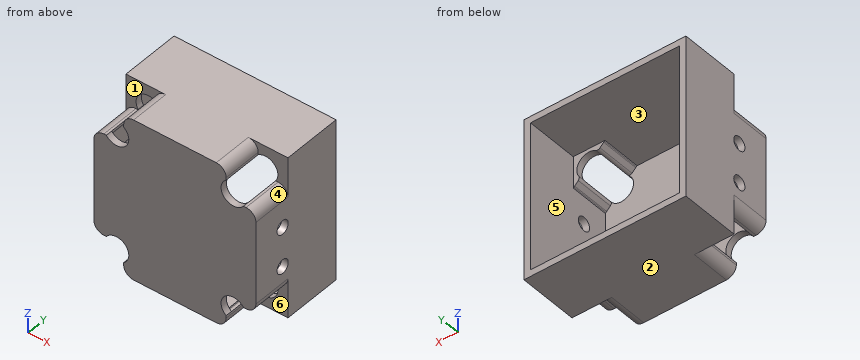
```python
from build123d import *

# Parameters (mm, degrees)
EXTRUDE_1_DEPTH          = 12
EXTRUDE_START            = 2
EXTRUDE_2_DEPTH          = 2
SKETCH_2_W               = 49
SKETCH_2_H               = 49
SKETCH_2_W_2             = 45
SKETCH_2_H_2             = 45
EXTRUDE_3_DEPTH          = 16
EXTRUDE_4_DEPTH          = 2
SKETCH_5_R               = 2.25
CUT_EXTRUDE_2_DEPTH      = 46.831212072
SKETCH_7_R               = 3.75
CUT_EXTRUDE_3_DEPTH      = 46.831212072
CUT_EXTRUDE_4_DEPTH      = 60.943723608
CUT_EXTRUDE_4_DEPTH_BACK = 60.943723608
SKETCH_8_R               = 2.1
CUT_EXTRUDE_10_DEPTH     = 12
FILLET_2_R               = 1


with BuildPart() as part:
    # 草图3 → 凸台-拉伸1 (new body)
    with BuildSketch(Plane(origin=(0, 0, 0), x_dir=(-1, 0, 0), z_dir=(0, -1, 0))):
        with BuildLine():
            Line((18.5, 15.5), (21.5, 15.5))
            ThreePointArc((21.5, 15.5), (23.621320344, 14.621320344), (24.5, 12.5))
            Line((24.5, 12.5), (24.5, -12.5))
            ThreePointArc((24.5, -12.5), (23.621320344, -14.621320344), (21.5, -15.5))
            Line((21.5, -15.5), (18.5, -15.5))
            ThreePointArc((18.5, -15.5), (16.378679656, -16.378679656), (15.5, -18.5))
            Line((15.5, -18.5), (15.5, -21.5))
            ThreePointArc((15.5, -21.5), (14.621320344, -23.621320344), (12.5, -24.5))
            Line((12.5, -24.5), (-12.5, -24.5))
            ThreePointArc((-12.5, -24.5), (-14.621320344, -23.621320344), (-15.5, -21.5))
            Line((-15.5, -21.5), (-15.5, -18.5))
            ThreePointArc((-15.5, -18.5), (-16.378679656, -16.378679656), (-18.5, -15.5))
            Line((-18.5, -15.5), (-21.5, -15.5))
            ThreePointArc((-21.5, -15.5), (-23.621320344, -14.621320344), (-24.5, -12.5))
            Line((-24.5, -12.5), (-24.5, 12.5))
            ThreePointArc((-24.5, 12.5), (-23.621320344, 14.621320344), (-21.5, 15.5))
            Line((-21.5, 15.5), (-18.5, 15.5))
            ThreePointArc((-18.5, 15.5), (-16.378679656, 16.378679656), (-15.5, 18.5))
            Line((-15.5, 18.5), (-15.5, 21.5))
            ThreePointArc((-15.5, 21.5), (-14.621320344, 23.621320344), (-12.5, 24.5))
            Line((-12.5, 24.5), (12.5, 24.5))
            ThreePointArc((12.5, 24.5), (14.621320344, 23.621320344), (15.5, 21.5))
            Line((15.5, 21.5), (15.5, 18.5))
            ThreePointArc((15.5, 18.5), (16.378679656, 16.378679656), (18.5, 15.5))
        make_face()
        with BuildLine():
            Line((18.5, 13.5), (21.5, 13.5))
            ThreePointArc((21.5, 13.5), (22.207106781, 13.207106781), (22.5, 12.5))
            Line((22.5, 12.5), (22.5, -12.5))
            ThreePointArc((22.5, -12.5), (22.207106781, -13.207106781), (21.5, -13.5))
            Line((21.5, -13.5), (18.5, -13.5))
            ThreePointArc((18.5, -13.5), (14.964466094, -14.964466094), (13.5, -18.5))
            Line((13.5, -18.5), (13.5, -21.5))
            ThreePointArc((13.5, -21.5), (13.207106781, -22.207106781), (12.5, -22.5))
            Line((12.5, -22.5), (-12.5, -22.5))
            ThreePointArc((-12.5, -22.5), (-13.207106781, -22.207106781), (-13.5, -21.5))
            Line((-13.5, -21.5), (-13.5, -18.5))
            ThreePointArc((-13.5, -18.5), (-14.964466094, -14.964466094), (-18.5, -13.5))
            Line((-18.5, -13.5), (-21.5, -13.5))
            ThreePointArc((-21.5, -13.5), (-22.207106781, -13.207106781), (-22.5, -12.5))
            Line((-22.5, -12.5), (-22.5, 12.5))
            ThreePointArc((-22.5, 12.5), (-22.207106781, 13.207106781), (-21.5, 13.5))
            Line((-21.5, 13.5), (-18.5, 13.5))
            ThreePointArc((-18.5, 13.5), (-14.964466094, 14.964466094), (-13.5, 18.5))
            Line((-13.5, 18.5), (-13.5, 21.5))
            ThreePointArc((-13.5, 21.5), (-13.207106781, 22.207106781), (-12.5, 22.5))
            Line((-12.5, 22.5), (12.5, 22.5))
            ThreePointArc((12.5, 22.5), (13.207106781, 22.207106781), (13.5, 21.5))
            Line((13.5, 21.5), (13.5, 18.5))
            ThreePointArc((13.5, 18.5), (14.964466094, 14.964466094), (18.5, 13.5))
        make_face(mode=Mode.SUBTRACT)
    extrude(amount=-EXTRUDE_1_DEPTH)

    # 草图4 → 凸台-拉伸2 (add)
    with BuildSketch(Plane.XZ.offset(EXTRUDE_START)):
        with BuildLine():
            Line((-24.5, 12.5), (-24.5, -12.5))
            ThreePointArc((-24.5, -12.5), (-23.621320344, -14.621320344), (-21.5, -15.5))
            Line((-21.5, -15.5), (-18.5, -15.5))
            ThreePointArc((-18.5, -15.5), (-16.378679656, -16.378679656), (-15.5, -18.5))
            Line((-15.5, -18.5), (-15.5, -21.5))
            ThreePointArc((-15.5, -21.5), (-14.621320344, -23.621320344), (-12.5, -24.5))
            Line((-12.5, -24.5), (12.5, -24.5))
            ThreePointArc((12.5, -24.5), (14.621320344, -23.621320344), (15.5, -21.5))
            Line((15.5, -21.5), (15.5, -18.5))
            ThreePointArc((15.5, -18.5), (16.378679656, -16.378679656), (18.5, -15.5))
            Line((18.5, -15.5), (21.5, -15.5))
            ThreePointArc((21.5, -15.5), (23.621320344, -14.621320344), (24.5, -12.5))
            Line((24.5, -12.5), (24.5, 12.5))
            ThreePointArc((24.5, 12.5), (23.621320344, 14.621320344), (21.5, 15.5))
            Line((21.5, 15.5), (18.5, 15.5))
            ThreePointArc((18.5, 15.5), (16.378679656, 16.378679656), (15.5, 18.5))
            Line((15.5, 18.5), (15.5, 21.5))
            ThreePointArc((15.5, 21.5), (14.621320344, 23.621320344), (12.5, 24.5))
            Line((12.5, 24.5), (-12.5, 24.5))
            ThreePointArc((-12.5, 24.5), (-14.621320344, 23.621320344), (-15.5, 21.5))
            Line((-15.5, 21.5), (-15.5, 18.5))
            ThreePointArc((-15.5, 18.5), (-16.378679656, 16.378679656), (-18.5, 15.5))
            Line((-18.5, 15.5), (-21.5, 15.5))
            ThreePointArc((-21.5, 15.5), (-23.621320344, 14.621320344), (-24.5, 12.5))
        make_face()
    extrude(amount=-EXTRUDE_2_DEPTH)

    # 草图2 → 凸台-拉伸3 (add)
    with BuildSketch(Plane(origin=(0, 12, 0), x_dir=(1, 0, 0), z_dir=(0, 1, 0))):
        Rectangle(SKETCH_2_W, SKETCH_2_H)
        Rectangle(SKETCH_2_W_2, SKETCH_2_H_2, mode=Mode.SUBTRACT)
    extrude(amount=EXTRUDE_3_DEPTH)

    # 草图6 → 凸台-拉伸4 (add)
    with BuildSketch(Plane.XZ.offset(-12).offset(EXTRUDE_START)):
        with BuildLine():
            Line((12.5, 24.5), (24.5, 24.5))
            Line((24.5, 24.5), (24.5, 12.5))
            ThreePointArc((24.5, 12.5), (23.621320344, 14.621320344), (21.5, 15.5))
            Line((21.5, 15.5), (18.5, 15.5))
            ThreePointArc((18.5, 15.5), (16.378679656, 16.378679656), (15.5, 18.5))
            Line((15.5, 18.5), (15.5, 21.5))
            ThreePointArc((15.5, 21.5), (14.621320344, 23.621320344), (12.5, 24.5))
        make_face()
        with BuildLine():
            Line((-24.5, -12.5), (-24.5, -24.5))
            Line((-24.5, -24.5), (-12.5, -24.5))
            ThreePointArc((-12.5, -24.5), (-14.621320344, -23.621320344), (-15.5, -21.5))
            Line((-15.5, -21.5), (-15.5, -18.5))
            ThreePointArc((-15.5, -18.5), (-16.378679656, -16.378679656), (-18.5, -15.5))
            Line((-18.5, -15.5), (-21.5, -15.5))
            ThreePointArc((-21.5, -15.5), (-23.621320344, -14.621320344), (-24.5, -12.5))
        make_face()
        with BuildLine():
            Line((-24.5, 12.5), (-24.5, 24.5))
            Line((-24.5, 24.5), (-12.5, 24.5))
            ThreePointArc((-12.5, 24.5), (-14.621320344, 23.621320344), (-15.5, 21.5))
            Line((-15.5, 21.5), (-15.5, 18.5))
            ThreePointArc((-15.5, 18.5), (-16.378679656, 16.378679656), (-18.5, 15.5))
            Line((-18.5, 15.5), (-21.5, 15.5))
            ThreePointArc((-21.5, 15.5), (-23.621320344, 14.621320344), (-24.5, 12.5))
        make_face()
        with BuildLine():
            Line((12.5, -24.5), (24.5, -24.5))
            Line((24.5, -24.5), (24.5, -12.5))
            ThreePointArc((24.5, -12.5), (23.621320344, -14.621320344), (21.5, -15.5))
            Line((21.5, -15.5), (18.5, -15.5))
            ThreePointArc((18.5, -15.5), (16.378679656, -16.378679656), (15.5, -18.5))
            Line((15.5, -18.5), (15.5, -21.5))
            ThreePointArc((15.5, -21.5), (14.621320344, -23.621320344), (12.5, -24.5))
        make_face()
    extrude(amount=-EXTRUDE_4_DEPTH)

    # 草图5 → 切除-拉伸2 (cut, through all)
    with BuildSketch(Plane.XZ.offset(2)):
        with Locations(Location((-17.7, 17.7, 0), (0, 0, 270))):
            Circle(SKETCH_5_R)
        with Locations(Location((-17.7, -17.7, 0), (0, 0, 270))):
            Circle(SKETCH_5_R)
        with Locations(Location((17.7, 17.7, 0), (0, 0, 270))):
            Circle(SKETCH_5_R)
        with Locations(Location((17.7, -17.7, 0), (0, 0, 270))):
            Circle(SKETCH_5_R)
    extrude(amount=-CUT_EXTRUDE_2_DEPTH, mode=Mode.SUBTRACT)

    # 草图7 → 切除-拉伸3 (cut, through all)
    with BuildSketch(Plane.XZ.offset(2)):
        with Locations(Location((-17.7, 17.7, 0), (0, 0, 270))):
            Circle(SKETCH_7_R)
        with Locations(Location((-17.7, -17.7, 0), (0, 0, 270))):
            Circle(SKETCH_7_R)
        with Locations(Location((17.7, -17.7, 0), (0, 0, 270))):
            Circle(SKETCH_7_R)
        with Locations(Location((17.7, 17.7, 0), (0, 0, 270))):
            Circle(SKETCH_7_R)
    extrude(amount=-CUT_EXTRUDE_3_DEPTH, mode=Mode.SUBTRACT)

    # 草图8 → 切除-拉伸4 (cut, two sides: drawn at the far end of the back side and taken through both)
    with BuildSketch(Plane.ZY.offset(-22.5).offset(-CUT_EXTRUDE_4_DEPTH_BACK)):
        with Locations((-7.5, 8)):
            Circle(SKETCH_8_R)
        with Locations((4.5, 8)):
            Circle(SKETCH_8_R)
    extrude(amount=CUT_EXTRUDE_4_DEPTH + CUT_EXTRUDE_4_DEPTH_BACK, mode=Mode.SUBTRACT)

    # 草图15 → 切除-拉伸10 (cut)
    with BuildSketch(Plane(origin=(0, 12, 0), x_dir=(1, 0, 0), z_dir=(0, 1, 0))):
        Polygon((-22.5, 12.9), (-22.5, -12.9), (-17.7, -17.7), (-12.9, -22.5), (12.9, -22.5), (17.7, -17.7), (22.5, -12.9), (22.5, 12.9), (17.7, 17.7), (12.9, 22.5), (-12.9, 22.5), (-17.7, 17.7), align=None)
    extrude(amount=-CUT_EXTRUDE_10_DEPTH, mode=Mode.SUBTRACT)

    # 圆角2
    # the kernel refuses this fillet: 1 mm, written as the material it takes off along each edge
    with BuildSketch(Plane(origin=(-15.048349571, 14.233859763, 20.351650429), x_dir=(-0.7779866052155301, 0, 0.6282808624375049), z_dir=(0, -1, 0))) as fillet_2_piece_1:
        with BuildLine():
            CenterArc((0.89979254, -0.994381263), FILLET_2_R, 96.076598735, 77.846802531)
            Line((-0.094588722, -0.888523317), (0, 0))
            ThreePointArc((0, 0), (0.396967297, -0.021070265), (0.793934594, 0))
        make_face()
    extrude(amount=14.233859763, mode=Mode.SUBTRACT)
    with BuildSketch(Plane(origin=(-20.351650429, 14.233859763, 15.048349571), x_dir=(-0.7071067811865058, 0, -0.7071067811865893), z_dir=(0, -1, 0)), Plane(origin=(-15.048349571, 14.233859763, -20.351650429), x_dir=(0.7071067811865506, 0, -0.7071067811865446), z_dir=(0, -1, 0))) as fillet_2_piece_2:
        with BuildLine():
            CenterArc((0.893543905, -1), FILLET_2_R, 90, 77.846802531)
            ThreePointArc((-0.084044285, -0.789473684), (-0.021070265, -0.396967297), (0, 0))
            Line((0, 0), (0.893543905, 0))
        make_face()
    extrude(amount=14.233859763, mode=Mode.SUBTRACT)
    with BuildSketch(Plane(origin=(20.351650429, 14.233859763, 15.048349571), x_dir=(0.7071067811864988, 0, -0.7071067811865962), z_dir=(0, -1, 0)), Plane(origin=(-20.351650429, 14.233859763, -15.048349571), x_dir=(-0.7071067811865525, 0, 0.7071067811865426), z_dir=(0, -1, 0)), Plane(origin=(15.048349571, 14.233859763, -20.351650429), x_dir=(-0.7071067811865416, 0, -0.7071067811865536), z_dir=(0, -1, 0))) as fillet_2_piece_3:
        with BuildLine():
            CenterArc((0.893543905, 1), FILLET_2_R, 192.153197469, 77.846802531)
            ThreePointArc((-0.084044285, 0.789473684), (-0.021070265, 0.396967297), (0, 0))
            Line((0, 0), (0.893543905, 0))
        make_face()
    extrude(amount=14.233859763, mode=Mode.SUBTRACT)
    with BuildSketch(Plane(origin=(15.048349571, 14.233859763, 20.351650429), x_dir=(0.7779866052154646, 0, 0.6282808624375861), z_dir=(0, -1, 0)), Plane(origin=(20.351650429, 14.233859763, -15.048349571), x_dir=(0.628280862437575, 0, -0.7779866052154735), z_dir=(0, -1, 0))) as fillet_2_piece_4:
        with BuildLine():
            CenterArc((0.89979254, 0.994381263), FILLET_2_R, 186.076598734, 77.846802531)
            Line((-0.094588722, 0.888523317), (0, 0))
            ThreePointArc((0, 0), (0.396967297, 0.021070265), (0.793934594, 0))
        make_face()
    extrude(amount=14.233859763, mode=Mode.SUBTRACT)


solid = part.part
```
Build history of the part. All positions in model axes, mm. Face numbers are marked on the shaded views. A direction names the side the tool comes from. Give positions to 0.01 mm unless a question says otherwise; leave off trailing zeros. Loops run counter-clockwise (first coordinate to the right, second up) from the corner with the lowest first, then second, coordinate; pieces in that order, holes last. Notation, with made-up numbers: (28, 24) -> (32, 24) arc R12 ccw to (32, 40) -> close; hole circle Ø3 at (-32.75, -4). An arc over 180 degrees is marked (long way). One line per question, with ' | ' between items.
Q1. Cut at A-A, the plane z = 4.5. Write the cut outline in (x, y).
Filled sheet:
outline: (-24.5, -2) -> (24.5, -2) -> (24.5, 5.9) -> (22.5, 5.9) -> (22.5, 0) -> (-22.5, 0) -> (-22.5, 5.9) -> (-24.5, 5.9) -> close; (-24.5, 10.1) -> (-22.5, 10.1) -> (-22.5, 28) -> (-24.5, 28) -> close; (22.5, 10.1) -> (24.5, 10.1) -> (24.5, 28) -> (22.5, 28) -> close
Q2. Drill centre lines: line 1 along Z through (x, y) = (-23.8, 8); line 2 along Z through (x, y) = (18, 26); line 3 along Y through (x, z) = (-23, 4.5). Where is each one in solid material? Low to high. Write a range as [from, to].
Filled sheet:
line 1: z = [-14.43, -9.6], [-5.4, 2.4], [6.6, 14.43] | line 2: z = [-24.5, -22.5], [22.5, 24.5] | line 3: y = [-2, 5.9], [10.1, 28]
Q3. Cut at D-D, the plane x = -4.5. Write the cut outline in (y, z), plus the area to 3 significant figures.
Filled sheet:
outline: (-2, -24.5) -> (28, -24.5) -> (28, -22.5) -> (0, -22.5) -> (0, 22.5) -> (28, 22.5) -> (28, 24.5) -> (-2, 24.5) -> close | area: 210 mm²
Q4. Tool access for the marked faces 4, 5 and 6: list every direction of +Z, -Z, +X, -X, +Y, -Y with a clear straight run to the whole face (end or side of a thin tool).
Filled sheet:
face 4: +Z, +X, -Y | face 5: +Y | face 6: -Z, +X, -Y
Q5. Cut at C-C, the plane x = -17.7. Write the cut outline in (y, z), plus the area to 3 significant figures.
Filled sheet:
outline: (-2, -13.95) -> (0, -13.95) -> (0, 13.95) -> (-2, 13.95) -> close; (10, -24.5) -> (28, -24.5) -> (28, -22.5) -> (12, -22.5) -> (12, -21.45) -> (10, -21.45) -> close; (10, 21.45) -> (12, 21.45) -> (12, 22.5) -> (28, 22.5) -> (28, 24.5) -> (10, 24.5) -> close | area: 132 mm²
Q6. Cut at B-B, the plane y = 23.5. Write the cut outline in (x, z), plus the area to 3 significant figures.
Filled sheet:
outline: (-24.5, -24.5) -> (24.5, -24.5) -> (24.5, 24.5) -> (-24.5, 24.5) -> close; hole (-22.5, -22.5) -> (22.5, -22.5) -> (22.5, 22.5) -> (-22.5, 22.5) -> close | area: 376 mm²
Q7. Drop flat-ended pins along their axis: pin 1 (6 mm diameter, centred on x = 19.5, z = 19.5, fed in from -Y); pin 2 (0.8 mm diameter, centred on y = 7, z = 21, fed in from +X); pin 3 (4 mm diameter, centred on x = -7.5, z = 0, fed in from +Y). Give the stop position or say it passes through.
Filled sheet:
pin 1: stops at y = 10 | pin 2: stops at x = 15.5 | pin 3: stops at y = 0
Q8. Pull direction Z, two halves, no side cores. Call the marked faces 1, 2 and 3: pulls with the +Z half, pulls with the -Z half, needs draft (parallel to the pull), parting line crosses it, or undercut.
Filled sheet:
face 1: needs draft | face 2: pulls with the -Z half | face 3: undercut
